Verification items for the finished model (mm, model axes). A direction names the side the tool comes from. Coordinates: 2 decimals unless noted, no trailing zeros. Order: outer loops, then holes, each group sorted by start corner. A loop starts at its lowest first (then second) coordinate and runs counter-clockwise, first axis right, second up. Notation, with made-up numbers: (6.25, -22) - (61.25, -22) arc R18 cw to (61.25, 12) - close; hole circle Ø10 at (30.25, 88). An arc over 180 degrees is marked (long way). Answer as CSV lines item,"result". Start each with the question number.
1. Material ranges on L1, parallel to Z at x = 109, y = 0.55; L2, parallel to X at y = 0.85, z = -41; L3, parallel to Y at x = 6, z = -37, recorded low to high. Write a range as [from, to].
2. Go/stop test with flat-tipped pins: pin 1 (2 mm diameter, centred on x = 66, y = 33, fed in from +Z); pin 2 (3 mm diameter, centred on x = 14.5, z = 2, fed in from +Y); pin 3 (0.6 mm diameter, centred on x = 34.5, y = 33.5, fed in from -Z); pin 4 (2 mm diameter, centred on y = 32.5, z = -17.5, fed in from -X). Record where each tip stops, or that it passes through.
3. Section check D-D (x = 47). Record the cut outline in (y, z), and give its area (3 significant figures).
4. Section check C-C (y = 9). Record the cut outline in (x, z).
5. Section check A-A (x = 109). Count the separate pieces of the cut face and the enclosed holes in it, and give its area (3 significant figures).
6. Mould release check, pull along Z, two halves, no side actions. Record for faces 5 (the flat face through (2, 2, -19)), 6 (the flat face through (42.6, 0, -37.6)): pulls with the +Z half, pulls with the -Z half, needs draft (parallel to the pull), parting line crosses it, or undercut.
7. Set-up check for faces 1 (the flat face through (120, 2, -19)), 2 (the flat face through (51, 3, -36)), 3 (the flat face through (110.4, 2, -39.6)), 4 (the flat face through (107.6, 2, 1.6)): record each of +Z, -Z, +X, -X, +Y, -Y from which the full face is reachable in a straight line by a thin tool's end or side.
from build123d import *

# Parameters (mm, degrees)
SKETCH1_W           = 122
SKETCH1_H           = 38
SKETCH1_W_2         = 118
SKETCH1_H_2         = 34
BOSS_EXTRUDE1_DEPTH = 34
SKETCH2_W           = 34
SKETCH2_H           = 2
BOSS_EXTRUDE2_DEPTH = 120
CUT_EXTRUDE2_DEPTH  = 2
SKETCH4_W           = 114
SKETCH4_H           = 26
CUT_EXTRUDE4_DEPTH  = 2
SKETCH6_W           = 114
SKETCH6_H           = 26
CUT_EXTRUDE5_DEPTH  = 2
SKETCH7_W           = 30
SKETCH7_H           = 26
CUT_EXTRUDE6_DEPTH  = 2
SKETCH8_W           = 12
SKETCH8_H           = 30
CUT_EXTRUDE7_DEPTH  = 2
LPATTERN1_COUNT     = 4
LPATTERN1_PITCH     = 16
SKETCH9_W           = 50
SKETCH9_H           = 30
CUT_EXTRUDE8_DEPTH  = 2
SKETCH10_W          = 6
SKETCH10_H          = 2
BOSS_EXTRUDE5_DEPTH = 6
SKETCH11_W          = 6
SKETCH11_H          = 2
BOSS_EXTRUDE6_DEPTH = 6
SKETCH12_W          = 6
SKETCH12_H          = 2
BOSS_EXTRUDE7_DEPTH = 6
SKETCH13_W          = 6
SKETCH13_H          = 2
BOSS_EXTRUDE8_DEPTH = 6
SKETCH14_R          = 1.5
CUT_EXTRUDE9_DEPTH  = 2


with BuildPart() as part:
    # Sketch1 → Boss-Extrude1 (new body)
    with BuildSketch(Plane(origin=(0, 0, 0), x_dir=(1, 0, 0), z_dir=(0, 1, 0))):
        with Locations((61, 19)):
            Rectangle(SKETCH1_W, SKETCH1_H)
        with Locations((61, 19)):
            Rectangle(SKETCH1_W_2, SKETCH1_H_2, mode=Mode.SUBTRACT)
    extrude(amount=BOSS_EXTRUDE1_DEPTH)

    # Sketch2 → Boss-Extrude2 (add)
    with BuildSketch(Plane.ZY):
        with Locations((-19, 33)):
            Rectangle(SKETCH2_W, SKETCH2_H)
    extrude(amount=-BOSS_EXTRUDE2_DEPTH)

    # Sketch3 → Cut-Extrude2 (cut)
    with BuildSketch(Plane.ZY):
        Polygon((-8, 2), (-2, 2), (-2, 15), (-4, 15), (-4, 19), (-2, 19), (-2, 32), (-11, 32), (-11, 30), (-27, 30), (-27, 32), (-36, 32), (-36, 19), (-34, 19), (-34, 15), (-36, 15), (-36, 2), (-30, 2), (-27, 2), (-27, 4), (-11, 4), (-11, 2), align=None)
    extrude(amount=-CUT_EXTRUDE2_DEPTH, mode=Mode.SUBTRACT)

    # Sketch4 → Cut-Extrude4 (cut)
    with BuildSketch(Plane(origin=(0, 0, -38), x_dir=(-1, 0, 0), z_dir=(0, 0, -1))):
        with Locations((-61, 17)):
            Rectangle(SKETCH4_W, SKETCH4_H)
    extrude(amount=-CUT_EXTRUDE4_DEPTH, mode=Mode.SUBTRACT)

    # Sketch6 → Cut-Extrude5 (cut)
    with BuildSketch(Plane.XY):
        with Locations((61, 17)):
            Rectangle(SKETCH6_W, SKETCH6_H)
    extrude(amount=-CUT_EXTRUDE5_DEPTH, mode=Mode.SUBTRACT)

    # Sketch7 → Cut-Extrude6 (cut)
    with BuildSketch(Plane(origin=(122, 0, 0), x_dir=(0, 0, -1), z_dir=(1, 0, 0))):
        with Locations((19, 17)):
            Rectangle(SKETCH7_W, SKETCH7_H)
    extrude(amount=-CUT_EXTRUDE6_DEPTH, mode=Mode.SUBTRACT)

    # Sketch8 → Cut-Extrude7 (cut)
    with BuildSketch(Plane(origin=(0, 34, 0), x_dir=(1, 0, 0), z_dir=(0, 1, 0))):
        with Locations((112, 19)):
            Rectangle(SKETCH8_W, SKETCH8_H)
    cut_extrude7 = extrude(amount=-CUT_EXTRUDE7_DEPTH, mode=Mode.SUBTRACT)

    # LPattern1: Cut-Extrude7 ×4
    with Locations(*[(-i * LPATTERN1_PITCH, 0, 0) for i in range(1, LPATTERN1_COUNT)]):
        add(cut_extrude7, mode=Mode.SUBTRACT)

    # Sketch9 → Cut-Extrude8 (cut)
    with BuildSketch(Plane(origin=(0, 34, 0), x_dir=(1, 0, 0), z_dir=(0, 1, 0))):
        with Locations((29, 19)):
            Rectangle(SKETCH9_W, SKETCH9_H)
    extrude(amount=-CUT_EXTRUDE8_DEPTH, mode=Mode.SUBTRACT)

    # Sketch10 → Boss-Extrude5 (add)
    with BuildSketch(Plane(origin=(0, 0, -38), x_dir=(-1, 0, 0), z_dir=(0, 0, -1))):
        with Locations((-13, 1)):
            Rectangle(SKETCH10_W, SKETCH10_H)
    extrude(amount=BOSS_EXTRUDE5_DEPTH)

    # Sketch11 → Boss-Extrude6 (add)
    with BuildSketch(Plane(origin=(0, 0, -38), x_dir=(-1, 0, 0), z_dir=(0, 0, -1))):
        with Locations((-109, 1)):
            Rectangle(SKETCH11_W, SKETCH11_H)
    extrude(amount=BOSS_EXTRUDE6_DEPTH)

    # Sketch12 → Boss-Extrude7 (add)
    with BuildSketch(Plane.XY):
        with Locations((13, 1)):
            Rectangle(SKETCH12_W, SKETCH12_H)
    extrude(amount=BOSS_EXTRUDE7_DEPTH)

    # Sketch13 → Boss-Extrude8 (add)
    with BuildSketch(Plane.XY):
        with Locations((109, 1)):
            Rectangle(SKETCH13_W, SKETCH13_H)
    extrude(amount=BOSS_EXTRUDE8_DEPTH)

    # Sketch14 → Cut-Extrude9 (cut)
    with BuildSketch(Plane.XZ):
        with Locations(Location((109, -41, 0), (0, 0, 270))):
            Circle(SKETCH14_R)
        with Locations(Location((109, 3, 0), (0, 0, 90))):
            Circle(SKETCH14_R)
        with Locations(Location((13, 3, 0), (0, 0, 270))):
            Circle(SKETCH14_R)
        with Locations(Location((13, -41, 0), (0, 0, 90))):
            Circle(SKETCH14_R)
    extrude(amount=-CUT_EXTRUDE9_DEPTH, mode=Mode.SUBTRACT)


solid = part.part
Evaluation:
1,L1,"z = [-44, -42.5], [-39.5, -36], [-2, 1.5], [4.5, 6]"
1,L2,"x = [10, 11.5], [14.5, 16], [106, 107.5], [110.5, 112]"
1,L3,"y = [0, 4], [30, 34]"
2,pin 1,"stops at z = 0"
2,pin 2,"stops at y = 2"
2,pin 3,"stops at z = -38"
2,pin 4,"stops at x = 0"
3,outline,"(0, -38) - (4, -38) - (4, -36) - (0, -36) - close; (0, -2) - (4, -2) - (4, 0) - (0, 0) - close; (30, -38) - (34, -38) - (34, -34) - (32, -34) - (32, -36) - (30, -36) - close; (30, -2) - (32, -2) - (32, -4) - (34, -4) - (34, 0) - (30, 0) - close"
3,area,"40.0 mm²"
4,outline,"(0, -38) - (4, -38) - (4, -36) - (0, -36) - close; (0, -2) - (4, -2) - (4, 0) - (0, 0) - close; (118, -38) - (122, -38) - (122, -34) - (120, -34) - (120, -36) - (118, -36) - close; (118, -2) - (120, -2) - (120, -4) - (122, -4) - (122, 0) - (118, 0) - close"
5,separate pieces,"6"
5,enclosed holes,"0"
5,area,"52.0 mm²"
6,face 5,"undercut"
6,face 6,"needs draft"
7,face 1,"-Y"
7,face 2,"none"
7,face 3,"-Z, +X, -X, +Y"
7,face 4,"+Z, +X, -X, +Y"
